Input: part model. Units: mm. Frame: model coordinates. Face numbers are marked on the shaded views. A direction names the side the tool comes from. Coordinates: 2 decimals unless noted, no trailing zeros. Loops run counter-clockwise (first coordinate to the right, second up) from the corner with the lowest first, then second, coordinate; pieces in that order, holes last.
```python
from build123d import *

# Parameters (mm, degrees)
F1_DEPTH = 73.1121525168
F2_R     = 26.6044020107
F3_DEPTH = 25.4


# Not quite as in the source:
# - the program builds the solid bodies; features that only make, move or delete a surface that nothing else refers to are left out


with BuildPart() as f1:
    # F0 (on Front) → F1 (new body)
    with BuildSketch(Plane.XZ):
        Polygon((-51.2930899858, 55.3425773978), (-49.3433475494, -37.4949574471), (47.5436300039, -37.4949574471), (47.5436300039, 55.3425773978), align=None)
    extrude(amount=F1_DEPTH)

    # F2 (on face) → F3 (join)
    with BuildSketch(Plane.XZ.offset(73.1121525168)):
        Circle(F2_R)
    extrude(amount=F3_DEPTH)


solid = f1.part
```
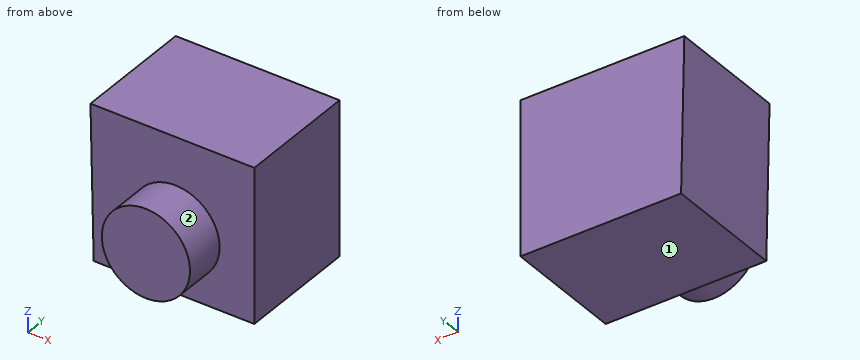
Item 1: Line query: L1, parallel to Y at x = 23.5, z = 42; L2, parallel to Z at x = 1, y = -91; L3, parallel to X at y = -34.5, z = -4. Output: solid intervals per line, ascending.
Result:
L1: y = -73.11 to 0
L2: z = -26.59 to 26.59
L3: x = -50.05 to 47.54
Item 2: Section query A-A (x = 0). Output: boundary loops of the cut face in (y, z).
Result:
outline: (-98.51, -26.6) - (-73.11, -26.6) - (-73.11, -37.49) - (0, -37.49) - (0, 55.34) - (-73.11, 55.34) - (-73.11, 26.6) - (-98.51, 26.6) - close
Item 3: Reachability of the marked faces 1 and 2 from +Z, -Z, +X, -X, +Y, -Y: full face, straight path, thin tool, end or side. Return the list, or none.
Result:
face 1: -Z, +X, -X, +Y, -Y
face 2: -Y
Item 4: Section query B-B (z = -20.5). Output: boundary loops of the cut face in (x, y), then the cut area to 3 significant figures.
Result:
outline: (-49.7, -73.11) - (-16.96, -73.11) - (-16.96, -98.51) - (16.96, -98.51) - (16.96, -73.11) - (47.54, -73.11) - (47.54, 0) - (-49.7, 0) - close
area: 7,970 mm2
Item 5: Section query D-D (x = -34). Output: boundary loops of the cut face in (y, z), then the cut area to 3 significant figures.
Result:
outline: (-73.11, -37.49) - (0, -37.49) - (0, 55.34) - (-73.11, 55.34) - close
area: 6,790 mm2
Item 6: Section query C-C (y = -91). Output: boundary loops of the cut face in (x, z).
Result:
outline: circle Ø53.21 at (0, 0)
Item 7: Contact query for flat-ended pins moving along their axis: P1, Ø2, axis at x = 3.5, y = -80, coming from the +Z side; P2, Ø2, axis at y = -53.5, z = 42, coming from the -X side; P3, Ø6, axis at x = -19.5, y = -85, coming from the -Z side; P4, Ø10, axis at x = -35, z = 20.5, coming from the +Y side. Output: stop coordinate, or through.
Result:
P1: stops at z = 26.49
P2: stops at x = -51.03
P3: stops at z = -20.87
P4: stops at y = 0
